The listing builds one solid part. Answer for the finished solid, in the listing's coordinates (mm). Face numbers are marked on the shaded views. A direction names the side the tool comes from. Give positions to 0.01 mm unless a question says otherwise; leave off trailing zeros. Order: outer loops, then holes, each group sorted by start corner. A loop starts at its lowest first (then second) coordinate and runs counter-clockwise, first axis right, second up. Notation, with made-up numbers: M 40.5,66 L 65.5,66 A26 cw 65.5,91 Z; hole C -13,26.5 d1. An arc over 180 degrees is marked long. Answer as a JSON object with one key per item and string values. Group by question number.
```python
from build123d import *

# Parameters (mm, degrees)
CIRPATTERN1_COUNT = 2
CIRPATTERN1_ANGLE = 90
THDSCHPAT_COUNT   = 15
THDSCHPAT_PITCH   = 0.635


with BuildPart() as part:
    # BodySke → Base-Revolve (revolve)
    with BuildSketch(Plane.XY, mode=Mode.PRIVATE) as base_revolve_sk:
        with BuildLine():
            Line((1.7272, 1.4224), (1.7272, 2.9845))
            Line((1.7272, 2.9845), (0.635, 2.888944882))
            ThreePointArc((0.635, 2.888944882), (0.160622478, 1.478954659), (0, 0))
            Line((0, 0), (11.2522, 0))
            Line((11.2522, 0), (11.2522, 1.4224))
            Line((11.2522, 1.4224), (1.7272, 1.4224))
        make_face()
    revolve(base_revolve_sk.sketch.rotate(Axis((-25.4, 0, 0), (1, 0, 0)), 90), axis=Axis((-25.4, 0, 0), (1, 0, 0)))

    # Sketch3 → Cross section 0
    with BuildSketch(Plane(origin=(0, 0, 0), x_dir=(0, 0, -1), z_dir=(1, 0, 0))):
        with BuildLine():
            Line((-0.4318, 1.9558), (0.4318, 1.9558))
            Line((0.4318, 1.9558), (0.4318, -1.9558))
            Line((0.4318, -1.9558), (-0.4318, -1.9558))
            Line((-0.4318, -1.9558), (-0.4318, 1.9558))
        make_face()
    # Sketch4 → Cross section 1
    with BuildSketch(Plane(origin=(2.1844, 0, 0), x_dir=(0, 0, -1), z_dir=(1, 0, 0))):
        with BuildLine():
            Line((-0.2159, 0.2159), (0.2159, 0.2159))
            Line((0.2159, 0.2159), (0.2159, -0.2159))
            Line((0.2159, -0.2159), (-0.2159, -0.2159))
            Line((-0.2159, -0.2159), (-0.2159, 0.2159))
        make_face()
    cross = loft(mode=Mode.SUBTRACT)

    # CirPattern1: Cross ×2 about axis
    cirpattern1_axis = Axis((0, 0, 0), (1, 0, 0))
    for i in range(1, CIRPATTERN1_COUNT):
        add(cross.rotate(cirpattern1_axis, i * CIRPATTERN1_ANGLE / (CIRPATTERN1_COUNT - 1)), mode=Mode.SUBTRACT)

    # ThdSchSke → ThreadSchematic (revolve, cut)
    with BuildSketch(Plane.XY):
        Polygon((2.3622, -1.04394), (2.097199455, -1.4224), (2.097199455, -1.778), (2.627200545, -1.778), (2.627200545, -1.4224), align=None)
    threadschematic = revolve(axis=Axis((-3.175, 0, 0), (1, 0, 0)), mode=Mode.SUBTRACT)

    # ThdSchPat: ThreadSchematic ×15
    with Locations(*[(i * THDSCHPAT_PITCH, 0, 0) for i in range(1, THDSCHPAT_COUNT)]):
        add(threadschematic, mode=Mode.SUBTRACT)


solid = part.part
```
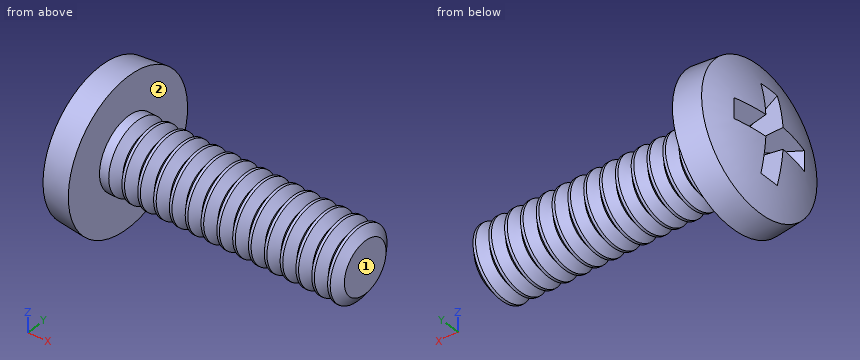
Item 1: Consider probe 1 along X at (y, z) = (1.5, 0.8); probe 2 along X at (y, z) = (1.2, -2); probe 3 along Z at (x, y) = (1.25, -2.15). Determine where each line is inside the solid, lowest interval first. Write a range as from..to.
Item 2: Flat-ended cylindrical pins translate along their axes: P1, Ø3, axis at x = 4.5, y = 0, coming from the +Z side; P2, Ø1.5, axis at y = 0, z = 1.5, coming from the +X side; P3, Ø3, axis at y = -2, z = -2, coming from the -X side; P4, Ø1, axis at y = 1, z = 2, coming from the -X side. Find the tip coordinate at first contact, or state that the pin passes through.
Item 3: Section A-A (x = 10.75) is taken. Determine the outline of the cut face in (y, z), and give its area (3 significant figures).
Item 4: A tool of negligible diameter and unlimited length cuts with its end or side. For the marked faces 1 and 2, from which of +Z, -Z, +X, -X, +Y, -Y can it reach the whole face along a straight path? Write none if from no direction.
Values found:
{
 "1": {"probe 1": "x = 0.21..1.73", "probe 2": "x = 0.41..1.73", "probe 3": "z = -2.01..2.01"},
 "2": {"P1": "stops at z = 1.42", "P2": "stops at x = 11.25", "P3": "stops at x = 0.13", "P4": "stops at x = 0.22"},
 "3": {"outline": "C 0,0 d2.47", "area": "4.78 mm^2"},
 "4": {"face 1": "+Z, -Z, +X, +Y, -Y", "face 2": "+X"}
}
